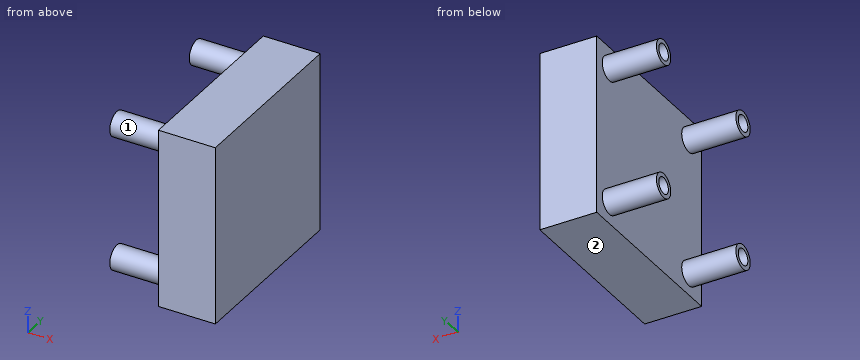
```python
from build123d import *

# Parameters (mm, degrees)
SKETCH1_W           = 33
SKETCH1_H           = 33
BOSS_EXTRUDE1_DEPTH = 10.5
SKETCH2_R           = 2.25
SKETCH2_R_2         = 1.5
BOSS_EXTRUDE2_DEPTH = 10


with BuildPart() as part:
    # Sketch1 → Boss-Extrude1 (new body)
    with BuildSketch(Plane(origin=(0, 0, 0), x_dir=(0, 0, -1), z_dir=(1, 0, 0))):
        Rectangle(SKETCH1_W, SKETCH1_H)
    extrude(amount=BOSS_EXTRUDE1_DEPTH)

    # Sketch2 → Boss-Extrude2 (add)
    # profile 1 of 4: a face of its own
    with BuildSketch(Plane.ZY):
        with Locations((-12.5, 12.5)):
            Circle(SKETCH2_R)
        with Locations((-12.5, 12.5)):
            Circle(SKETCH2_R_2, mode=Mode.SUBTRACT)
    # profile 2 of 4: a face of its own
    with BuildSketch(Plane.ZY):
        with Locations((-12.5, -12.5)):
            Circle(SKETCH2_R)
        with Locations((-12.5, -12.5)):
            Circle(SKETCH2_R_2, mode=Mode.SUBTRACT)
    # profile 3 of 4: a face of its own
    with BuildSketch(Plane.ZY):
        with Locations((12.5, -12.5)):
            Circle(SKETCH2_R)
        with Locations((12.5, -12.5)):
            Circle(SKETCH2_R_2, mode=Mode.SUBTRACT)
    # profile 4 of 4: a face of its own
    with BuildSketch(Plane.ZY):
        with Locations((12.5, 12.5)):
            Circle(SKETCH2_R)
        with Locations((12.5, 12.5)):
            Circle(SKETCH2_R_2, mode=Mode.SUBTRACT)
    extrude(amount=BOSS_EXTRUDE2_DEPTH)


solid = part.part
```
CAD build for the part. Positions are in the model's coordinates, mm. Face numbers are marked on the shaded views. A direction names the side the tool comes from. Round coordinates to 2 decimals unless told otherwise and drop trailing zeros. Write each loop counter-clockwise with the first axis right and the second up, starting at its lowest first coordinate (ties: lowest second). Pieces come first, ordered by that corner, then holes. Notation, with made-up numbers: (-38.5, 65) - (16.5, 65) arc R20 ccw to (16.5, 99) - close; hole circle Ø1 at (75, -11.5). An arc over 180 degrees is marked (long way). Return JSON: item names as keys, results as strings. Group by question number.
Item 1: Probe probe 1 along Y at (x, z) = (-5.5, -12.5); probe 2 along Y at (x, z) = (-3.5, 13); probe 3 along X at (y, z) = (12, 7). List the from-to ranges inside material, lowest first.
Item 2: 3-axis set-ups, long thin cutter, end or side, ignore diameter. For the marked faces 1 and 2: which of +Z, -Z, +X, -X, +Y, -Y reach the whole face in a straight line?
Item 3: Band-saw the part on A-A on x = -6.75. List the corners of the cut face in (y, z), plus the area to 3 significant figures.
Item 4: Band-saw the part on D-D on y = 2. List the corners of the cut face in (x, z).
Item 5: Flat gauge pins, fed straight in: pin 1 Ø2.5 at (y, z) = (-12.5, 12.5) entering from -X; pin 2 Ø4 at (x, z) = (-3.5, 12.5) entering from +Y. Where does each tip first touch, or does it go through?
Item 6: Band-saw the part on B-B on y = -12.5. List the corners of the cut face in (x, z), plus the area to 4 significant figures.
Resolved:
{
 "1": {"probe 1": "y = -14.75 to -14, -11 to -10.25, 10.25 to 11, 14 to 14.75", "probe 2": "y = -14.69 to -13.91, -11.09 to -10.31, 10.31 to 11.09, 13.91 to 14.69", "probe 3": "x = 0 to 10.5"},
 "2": {"face 1": "-X", "face 2": "-Z, +X, -X, +Y, -Y"},
 "3": {"outline": "circle Ø4.5 at (-12.5, -12.5); circle Ø4.5 at (-12.5, 12.5); circle Ø4.5 at (12.5, -12.5); circle Ø4.5 at (12.5, 12.5); hole circle Ø3 at (-12.5, -12.5); hole circle Ø3 at (-12.5, 12.5); hole circle Ø3 at (12.5, -12.5); hole circle Ø3 at (12.5, 12.5)", "area": "35.3 mm²"},
 "4": {"outline": "(0, -16.5) - (10.5, -16.5) - (10.5, 16.5) - (0, 16.5) - close"},
 "5": {"pin 1": "stops at x = 0", "pin 2": "stops at y = 14.75"},
 "6": {"outline": "(-10, -14.75) - (0, -14.75) - (0, -16.5) - (10.5, -16.5) - (10.5, 16.5) - (0, 16.5) - (0, 14.75) - (-10, 14.75) - (-10, 14) - (0, 14) - (0, 11) - (-10, 11) - (-10, 10.25) - (0, 10.25) - (0, -10.25) - (-10, -10.25) - (-10, -11) - (0, -11) - (0, -14) - (-10, -14) - close", "area": "376.5 mm²"}
}
